Autodesk Inventor part; units mm, degrees
ref_plane "YZ Plane" through (0, 0, 0) normal (1, 0, 0) x (0, 1, 0)
ref_plane "XZ Plane" through (0, 0, 0) normal (0, 1, 0) x (-1, 0, 0)
ref_plane "XY Plane" through (0, 0, 0) normal (0, 0, 1) x (1, 0, 0)
sketch "Sketch1" plane through (0, 0, 0) normal (0, 1, 0) x (-1, 0, 0)
  point P0 (0, 0)
sketch "Sketch2" plane through (0, 0, 0) normal (0, 1, 0) x (-1, 0, 0)
  line L0 (0, 0) -> (-50, 0)
  line L1 (-50, 0) -> (-50, -50)
  line L2 (-50, -50) -> (0, -50)
  line L3 (0, -50) -> (0, 0)
  line L4 (0, -25) -> (-11.3835, -25)
  line L5 (-25, -50) -> (-25, 0)
  circle A0 centre (-7.5, -42.5) radius 2
  circle A1 centre (-7.5, -7.5) radius 2
  line L6 (-7.5, -42.5) -> (-7.5, -50)
  line L7 (-7.5, -7.5) -> (-7.5, 0)
  line L8 (-7.5, -42.5) -> (0, -42.5)
  line L9 (-10, -27) -> (-14, -27)
  line L10 (-14, -27) -> (-14, -23)
  line L11 (-14, -23) -> (-10, -23)
  line L12 (-10, -23) -> (-10, -27)
  circle A2 centre (-42.5, -42.5) radius 2
  circle A3 centre (-42.5, -7.5) radius 2
  line L13 (-40, -27) -> (-36, -27)
  line L14 (-36, -27) -> (-36, -23)
  line L15 (-36, -23) -> (-40, -23)
  line L16 (-40, -23) -> (-40, -27)
  circle A4 centre (-25, -25) radius 2
  line L17 (-14, -27) -> (-14, -30)
  line L18 (-14, -30) -> (-30, -30)
  line L19 (-30, -30) -> (-30, -37)
  line L20 (-30, -37) -> (-10, -37)
  line L21 (-10, -37) -> (-10, -27)
  line L22 (-40, -23) -> (-40, -13)
  line L23 (-40, -13) -> (-20, -13)
  line L24 (-20, -13) -> (-20, -20)
  line L25 (-20, -20) -> (-36, -20)
  line L26 (-36, -20) -> (-36, -23)
  line L27 (-30, -33.5) -> (-10, -33.5)
  line L28 (-20, -16.5) -> (-40, -16.5)
  circle A5 centre (-25, -33.5) radius 2
  circle A6 centre (-15, -33.5) radius 2
  circle A7 centre (-25, -16.5) radius 2
  circle A8 centre (-35, -16.5) radius 2
  point P0 (-10, -25)
  point P1 (-40, -25)
  dimension "d0" = 50
  dimension "d1" = 4
  dimension "d2" = 35
  dimension "d6" = 4
  dimension "d7" = 10
  dimension "d8" = 4
  dimension "d9" = 10
  dimension "d10" = 7
  dimension "d11" = 20
  dimension "d12" = 10
  dimension "d13" = 10
  dimension "d14" = 4
  dimension "d15" = 4
  dimension "d16" = 4
  dimension "d17" = 4
extrude "Extrusion1" add sketch "Sketch2" along normal blind 10 contours L3 L4 L12 L11 L10 L17 L18 L5 A4 L25 L24 L23 L0 | L3 L8 A0 L6 L2 L5 L20 L21 L12 L4 | L5 L23 L22 L16 L13 L14 L26 L25 A4 L18 L19 L20 L2 L1 L0 | L3 L2 L6 A0 L8
extrude "Extrusion2" add sketch "Sketch2" along normal blind 5 contours L23 L24 L28 A7 L5 | L5 A7 L28 A8 L22 L23 | L21 L27 A6 A5 L5 L18 L17 L9 | L21 L20 L5 A5 L27 A6 | L28 L24 L25 L5 A7 | A7 L5 L25 L26 L15 L22 L28 A8 | L20 L19 L27 A5 L5 | L5 A5 L27 L19 L18
fillet "Fillet1" radius 2 2 edges at (12, 5, -27) (38, 5, -23)
equation "\"d0\" = width"
equation "\"d1\" = screw_hole_diameter"
equation "\"d2\" = hole_spacing"
equation "\"d6\" = cabel_channel_depth"
equation "\"d8\" = screw_hole_diameter"
equation "\"d18\" = plate_thicknes"
equation "\"d20\" = 0.5 * plate_thicknes"
equation "\"plate_thicknes\" = 10"
properties part number "2_inner_leg_top_plate"
CAD build for the part. Positions are in the model's coordinates, mm. A direction names the side the tool comes from. Round coordinates to 2 decimals unless told otherwise and drop trailing zeros. Loops run counter-clockwise (first coordinate to the right, second up) from the corner with the lowest first, then second, coordinate; pieces in that order, holes last. Notation, with made-up numbers: (64, -34.75) - (85, -34.75) arc R28 ccw to (85, -14.75) - close; hole circle Ø3 at (-40, 45). An arc over 180 degrees is marked (long way). Return JSON: item names as keys, results as strings. Group by question number.
Q1. Band-saw the part on A-A on z = -33.5. Give the cut face in (x, y).
Q2. Band-saw the part on C-C on x = 7.5. Give the cut face in (y, z), plus the area to 3 significant figures.
Q3. Band-saw the part on D-D on z = -25. Give the cut face in (x, y).
Q4. Drill centre lines: line 1 along Z through (x, y) = (25, 2.85); line 2 along X through (y, z) = (5.25, -25); line 3 along X through (y, z) = (2.7, -33.5). Where is each one in solid material? Low to high. Write a range as [from, to].
Q5. Band-saw the part on B-B on x = 15. Give the cut face in (y, z).
Q6. Tool access for faces 4 (the face through (30, 7, -33)), 5 (the face through (12, 1, -27)): list every direction of +Z, -Z, +X, -X, +Y, -Y with a clear straight run to the whole face (end or side of a thin tool).
Q7. Two-plate mould, pull along Z, no slides. Class faces 1 (the face through (25, 5, -50)), 2 (the face through (8.974, 4.93, -8.852)), 3 (the face through (0, 5, -25)): +Z half, -Z half, draft (parallel to the pull), parting line (faces both ways), or undercut.
Solutions:
{
 "1": {"outline": "(0, 0) - (13, 0) - (13, 5) - (10, 5) - (10, 10) - (0, 10) - close; (17, 0) - (23, 0) - (23, 5) - (17, 5) - close; (27, 0) - (50, 0) - (50, 10) - (30, 10) - (30, 5) - (27, 5) - close"},
 "2": {"outline": "(0, -50) - (10, -50) - (10, -44.5) - (0, -44.5) - close; (0, -40.5) - (10, -40.5) - (10, -9.5) - (0, -9.5) - close; (0, -5.5) - (10, -5.5) - (10, 0) - (0, 0) - close", "area": "420 mm^2"},
 "3": {"outline": "(0, 0) - (10, 0) - (10, 10) - (0, 10) - close; (14, 0) - (23, 0) - (23, 10) - (14, 10) - close; (27, 0) - (36, 0) - (36, 10) - (27, 10) - close; (40, 0) - (50, 0) - (50, 10) - (40, 10) - close"},
 "4": {"line 1": "z = [-50, -35.5], [-31.5, -27], [-23, -18.5], [-14.5, 0]", "line 2": "x = [0, 10], [14, 23], [27, 36], [40, 50]", "line 3": "x = [0, 13], [17, 23], [27, 50]"},
 "5": {"outline": "(0, -50) - (10, -50) - (10, -37) - (5, -37) - (5, -35.5) - (0, -35.5) - close; (0, -31.5) - (5, -31.5) - (5, -30) - (10, -30) - (10, 0) - (0, 0) - close"},
 "6": {"face 4": "+Y", "face 5": "+Y, -Y"},
 "7": {"face 1": "-Z half", "face 2": "undercut", "face 3": "draft"}
}
